from build123d import *

# Parameters (mm, degrees)
BOSS_EXTRU_1_DEPTH      = 4
ESQUISSE2_R             = 3.75
BOSS_EXTRU_2_DEPTH      = 5.5
ESQUISSE3_R             = 2.5
BOSS_EXTRU_3_DEPTH      = 2
ENL_V_MAT_EXTRU_2_DEPTH = 30.955633861
BOSS_EXTRU_7_DEPTH      = 4.5
ESQUISSE7_R             = 0.75
ENL_V_MAT_EXTRU_3_DEPTH = 8
ESQUISSE8_W             = 30
ESQUISSE8_H             = 4
BOSS_EXTRU_8_DEPTH      = 5.5
ESQUISSE9_W             = 30
ESQUISSE9_H             = 2.5
BOSS_EXTRU_9_DEPTH      = 10
ESQUISSE10_R            = 2.05
ENL_V_MAT_EXTRU_4_DEPTH = 37.43267764
CONG_2_R                = 1.5


with BuildPart() as part:
    # Esquisse1 → Boss.-Extru.1 (new body)
    with BuildSketch(Plane(origin=(0, 0, 0), x_dir=(1, 0, 0), z_dir=(0, 1, 0))):
        with BuildLine():
            Line((-15, 10.998181668), (-15, 16.5))
            Line((-15, 16.5), (15, 16.5))
            Line((15, 16.5), (15, 10.998181668))
            ThreePointArc((15, 10.998181668), (21.946875755, -2.451715724), (10.2, -12))
            Line((10.2, -12), (-10.2, -12))
            ThreePointArc((-10.2, -12), (-21.946875755, -2.451715724), (-15, 10.998181668))
        make_face()
    extrude(amount=BOSS_EXTRU_1_DEPTH)

    # Esquisse2 → Boss.-Extru.2 (add)
    with BuildSketch(Plane.XZ):
        with Locations(Location((-10.2, 0, 0), (0, 0, 90))):
            Circle(ESQUISSE2_R)
    extrude(amount=BOSS_EXTRU_2_DEPTH)

    # Esquisse3 → Boss.-Extru.3 (add)
    with BuildSketch(Plane.XZ.offset(5.5)):
        with Locations(Location((-10.2, 0, 0), (0, 0, 270))):
            Circle(ESQUISSE3_R)
    extrude(amount=BOSS_EXTRU_3_DEPTH)

    # Esquisse5 → Enlèv. mat.-Extru.2 (cut, through all)
    with BuildSketch(Plane(origin=(0, 4, 0), x_dir=(1, 0, 0), z_dir=(0, 1, 0))):
        with BuildLine():
            ThreePointArc((4.95, 2.90473751), (16.2, 0), (4.95, -2.90473751))
            ThreePointArc((4.95, -2.90473751), (1.2, 0), (4.95, 2.90473751))
        make_face()
    extrude(amount=-ENL_V_MAT_EXTRU_2_DEPTH, mode=Mode.SUBTRACT)

    # Esquisse6 → Boss.-Extru.7 (add)
    with BuildSketch(Plane(origin=(0, 4, 0), x_dir=(1, 0, 0), z_dir=(0, 1, 0))):
        with BuildLine():
            ThreePointArc((18.670537173, -8.5), (22.2, 0), (18.670537173, 8.5))
            Line((18.670537173, 8.5), (-11.8, 8.5))
            ThreePointArc((-11.8, 8.5), (-13.214213562, 7.914213562), (-13.8, 6.5))
            Line((-13.8, 6.5), (-13.8, -6.5))
            ThreePointArc((-13.8, -6.5), (-13.214213562, -7.914213562), (-11.8, -8.5))
            Line((-11.8, -8.5), (18.670537173, -8.5))
        make_face()
        Polygon((16.2, 0), (16.2, -6), (10.2, -6), (-6.8, -6), (-6.8, 6), (10.2, 6), (16.2, 6), align=None, mode=Mode.SUBTRACT)
    extrude(amount=BOSS_EXTRU_7_DEPTH)

    # Esquisse7 → Enlèv. mat.-Extru.3 (cut)
    with BuildSketch(Plane(origin=(0, 8.5, 0), x_dir=(1, 0, 0), z_dir=(0, 1, 0))):
        with BuildLine():
            ThreePointArc((-10.05, 0), (-9.3, -0.75), (-8.55, 0))
            Line((-8.55, 0), (-10.05, 0))
        make_face()
        with BuildLine():
            Line((-10.05, 0), (-8.55, 0))
            ThreePointArc((-8.55, 0), (-9.3, 0.75), (-10.05, 0))
        make_face()
        with Locations(Location((18.7, 0, 0), (0, 0, 270))):
            Circle(ESQUISSE7_R)
    extrude(amount=-ENL_V_MAT_EXTRU_3_DEPTH, mode=Mode.SUBTRACT)

    # Esquisse8 → Boss.-Extru.8 (add)
    with BuildSketch(Plane.XZ):
        with Locations((0, -14.5)):
            Rectangle(ESQUISSE8_W, ESQUISSE8_H)
    extrude(amount=BOSS_EXTRU_8_DEPTH)

    # Esquisse9 → Boss.-Extru.9 (add)
    with BuildSketch(Plane(origin=(0, 0, -16.5), x_dir=(-1, 0, 0), z_dir=(0, 0, -1))):
        with Locations((0, -4.25)):
            Rectangle(ESQUISSE9_W, ESQUISSE9_H)
    extrude(amount=BOSS_EXTRU_9_DEPTH)

    # Esquisse10 → Enlèv. mat.-Extru.4 (cut, through all)
    with BuildSketch(Plane(origin=(0, -3, 0), x_dir=(1, 0, 0), z_dir=(0, 1, 0))):
        with Locations(Location((-8, 21.5, 0), (0, 0, 270))):
            Circle(ESQUISSE10_R)
        with Locations(Location((8, 21.5, 0), (0, 0, 90))):
            Circle(ESQUISSE10_R)
    extrude(amount=-ENL_V_MAT_EXTRU_4_DEPTH, mode=Mode.SUBTRACT)

    # Congé2
    cong_2_edges = [part.edges().sort_by_distance(p)[0] for p in [
        (0, 4, -16.5),
    ]]
    fillet(cong_2_edges, radius=CONG_2_R)


solid = part.part
Geometry check sheet. Reference: the model listing, model coordinates, mm. A direction names the side the tool comes from. Give positions to 0.01 mm unless a question says otherwise; leave off trailing zeros. Order: outer loops, then holes, each group sorted by start corner. A loop starts at its lowest first (then second) coordinate and runs counter-clockwise, first axis right, second up. Notation, with made-up numbers: (47.5, -9.5) - (52.5, -9.5) arc R10 ccw to (52.5, 5.5) - close; hole circle Ø8 at (-15, 44). An arc over 180 degrees is marked (long way). Use one line per item in the form item = value.
1) Depth check by flat-ended pin: pin 1 Ø2 at (x, y) = (8, 7) entering from +Z; pin 2 Ø3 at (x, z) = (14.5, -2.5) entering from +Y; pin 3 Ø1.4 at (x, z) = (18.7, 0) entering from -Y. Enter the tip coordinate at first touch or a pass-through.
Working result:
pin_1 = 8.5
pin_2 = 4
pin_3 = 0
2) Material ranges on probe 1 along X at (y, z) = (-3.55, -21.5); probe 2 along X at (y, z) = (4.25, 0); probe 3 along Z at (x, y) = (14, 4.25), recorded low to high. Write a range as from..to.
Working result:
probe_1 = -15..-10.05, -5.95..5.95, 10.05..15
probe_2 = -13.8..-10.05, -8.55..-6.8, 16.2..17.95, 19.45..22.2
probe_3 = -8.5..-6, 6..8.5
3) Sectioned sample at C-C (y = 5.75). Record the boundary of the cut face in (x, z).
Working result:
outline = (-13.8, -6.5) arc R2 ccw to (-11.8, -8.5) - (18.67, -8.5) arc R12 ccw to (18.67, 8.5) - (-11.8, 8.5) arc R2 ccw to (-13.8, 6.5) - close; hole circle Ø1.5 at (-9.3, 0); hole (-6.8, -6) - (16.2, -6) - (16.2, 6) - (-6.8, 6) - close; hole circle Ø1.5 at (18.7, 0)
4) Sectioned sample at D-D (x = 8). Record the boundary of the cut face in (y, z), and give its area (3 significant figures).
Working result:
outline = (-5.5, -26.5) - (-3, -26.5) - (-3, -23.55) - (-5.5, -23.55) - close; (-5.5, -19.45) - (-3, -19.45) - (-3, -16.5) - (2.5, -16.5) arc R1.5 ccw to (4, -15) - (4, -8.5) - (8.5, -8.5) - (8.5, -6) - (4, -6) - (4, -5.58) - (0, -5.58) - (0, -12.5) - (-5.5, -12.5) - close; (0, 5.58) - (4, 5.58) - (4, 6) - (8.5, 6) - (8.5, 8.5) - (4, 8.5) - (4, 12) - (0, 12) - close
area = 128 mm^2
5) Draft check along Z on faces 1 (the face through (0, -5.5, -19)), 2 (the face through (5, 6, -6)), 3 (the face through (-21.898, 1.972, 2.676)), 4 (the face through (-13.2, 6.22, -7.93)). Enter one of: released by +Z, released by -Z, zero draft, split by the parting line, or undercut.
Working result:
face_1 = zero draft
face_2 = undercut
face_3 = split by the parting line
face_4 = released by -Z
6) Sectioned sample at A-A (y = -3.5). Record the boundary of the cut face in (x, z), and give its area (3 significant figures).
Working result:
outline = (-15, -26.5) - (15, -26.5) - (15, -12.5) - (-15, -12.5) - close; circle Ø7.5 at (-10.2, 0); hole circle Ø4.1 at (-8, -21.5); hole circle Ø4.1 at (8, -21.5)
area = 438 mm^2
7) Sectioned sample at B-B (x = -0.5). Record the boundary of the cut face in (y, z), and give its area (3 significant figures).
Working result:
outline = (-5.5, -26.5) - (-3, -26.5) - (-3, -16.5) - (2.5, -16.5) arc R1.5 ccw to (4, -15) - (4, -8.5) - (8.5, -8.5) - (8.5, -6) - (4, -6) - (4, 6) - (8.5, 6) - (8.5, 8.5) - (4, 8.5) - (4, 12) - (0, 12) - (0, -12.5) - (-5.5, -12.5) - close
area = 183 mm^2
8) Access from +Z, -Z, +X, -X, +Y, -Y to the whole of each face (thin tool, end or side, straight path). Record for faces 5 (the face through (15, -2, -15)), 6 (the face through (0, -3, -12.5)), 7 (the face through (-13.8, 6, 0)).
Working result:
face_5 = -Z, +X, +Y, -Y
face_6 = +X, -X, -Y
face_7 = +Z, -Z, -X, +Y
